Geometry check sheet. Reference: the model listing, model coordinates, mm. Coordinates: 2 decimals unless noted, no trailing zeros. Order: outer loops, then holes, each group sorted by start corner. A loop starts at its lowest first (then second) coordinate and runs counter-clockwise, first axis right, second up. Notation, with made-up numbers: (-38.75, 50.25) - (-12.75, 50.25) arc R26 cw to (-12.75, 87.25) - close; hole circle Ø4 at (84.5, 45.5). An arc over 180 degrees is marked (long way). Use CSV: the item, a comma, the result in double quotes. Start each with the question number.
1) Sectioned sample at A-A, the plane y = 147.5. Count the separate pieces of the cut face and the enclosed holes in it, and give its area (3 significant figures).
2) Depth check by flat-ended pin: P1, Ø3, axis at y = 143.5, z = -33.5, coming from the +X side. Enter the tip coordinate at first touch or a pass-through.
3) Thickness scan on probe 1 along Z at (x, y) = (189, 83); probe 2 along X at (y, z) = (158.5, -37). Record the ranges inside material, lowest first. Write a range as [from, to].
4) Sectioned sample at B-B, the plane z = -27. Record the cut outline in (x, y).
from build123d import *

# Parameters (mm, degrees)
SKETCH1_R           = 3.3782
SKETCH1_R_2         = 2.5
BOSS_EXTRUDE1_DEPTH = 203.2


with BuildPart() as part:
    # Sketch1 → Boss-Extrude1 (new body)
    with BuildSketch(Plane(origin=(0, 0, 0), x_dir=(1, 0, 0), z_dir=(0, 1, 0))):
        with BuildLine():
            Line((-205.948559195, -52.784375), (205.948559195, -52.784375))
            Line((205.948559195, -52.784375), (205.948559195, 7.252981651))
            ThreePointArc((205.948559195, 7.252981651), (205.62400269, 9.718233056), (204.672451166, 12.015481651))
            Line((204.672451166, 12.015481651), (181.134519617, 52.784375))
            Line((181.134519617, 52.784375), (-205.948559195, 52.784375))
            Line((-205.948559195, 52.784375), (-205.948559195, -52.784375))
        make_face()
        with Locations(Location((-196.423559195, 43.259375, 0), (0, 0, 270))):
            Circle(SKETCH1_R, mode=Mode.SUBTRACT)
        with Locations(Location((-196.423559195, -43.259375, 0), (0, 0, 270))):
            Circle(SKETCH1_R, mode=Mode.SUBTRACT)
        with Locations(Location((196.423559195, 7.252981651, 0), (0, 0, 270))):
            Circle(SKETCH1_R, mode=Mode.SUBTRACT)
        with Locations(Location((174.198559195, 33.3375, 0), (0, 0, 270))):
            Circle(SKETCH1_R_2, mode=Mode.SUBTRACT)
        with Locations(Location((-38.526440805, 33.3375, 0), (0, 0, 270))):
            Circle(SKETCH1_R_2, mode=Mode.SUBTRACT)
        with Locations(Location((-38.526440805, -33.3375, 0), (0, 0, 90))):
            Circle(SKETCH1_R_2, mode=Mode.SUBTRACT)
        with Locations(Location((174.198559195, -33.3375, 0), (0, 0, 90))):
            Circle(SKETCH1_R_2, mode=Mode.SUBTRACT)
    extrude(amount=BOSS_EXTRUDE1_DEPTH)


solid = part.part
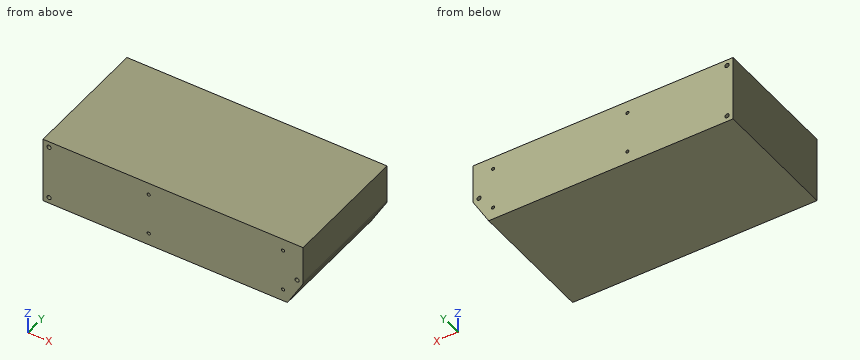
Evaluation:
1,separate pieces,"1"
1,enclosed holes,"7"
1,area,"42,800 mm²"
2,P1,"x = 193.13"
3,probe 1,"[-39.16, 52.78]"
3,probe 2,"[-205.95, 190.25]"
4,outline,"(-205.95, 0) - (196.02, 0) - (196.02, 203.2) - (-205.95, 203.2) - close"
